Source: three-view drawing plus pictorial views. Frame: mm from the lowest corner of the part. Coordinates: 2 decimals unless noted, no trailing zeros. Order: outer loops, then holes, each group sorted by start corner. A loop starts at its lowest first (then second) coordinate and runs counter-clockwise, first axis right, second up. Notation, with made-up numbers: M 30.25,11 L 64.25,11 A18 cw 64.25,20 Z; hole C -17.75,-7 d4. An arc over 180 degrees is marked long. Use CSV: the item, a comma, the result in double quotes. Start each with the question number.
Q1. Section query A-A, the plane z = 11.5. State how many separate pieces and enclosed holes the cut face has, and give its area (3 significant figures).
Q2. Ray query, probe 1 along Y at (x, z) = (62, 16.75); probe 2 along Z at (x, y) = (37, 114). Return the intervals inside material, ascending.
Q3. Section query B-B, the plane x = 69. Output: boundary loops of the cut face in (y, z), and give its area (3 significant figures).
Q4. First-contact query: P1, Ø8, axis at x = 58, y = 24, coming from the +Z side; P2, Ø8, axis at y = 30, z = 8, coming from the -X side. Flat tips, straight axial feed; report the tip coordinate or a pass-through.
Q5. Section query C-C, the plane y = 60. Output: boundary loops of the cut face in (x, z).
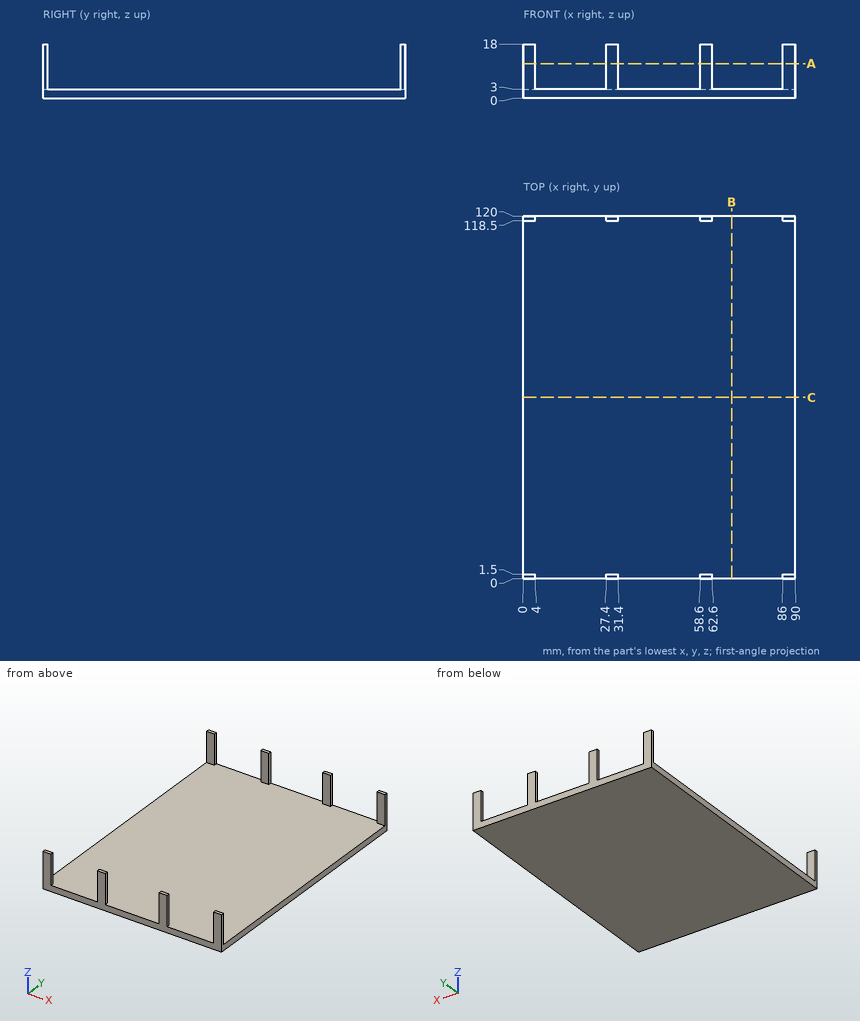
Responses:
1,separate pieces,"8"
1,enclosed holes,"0"
1,area,"48.0 mm²"
2,probe 1,"y = 0 to 1.5, 118.5 to 120"
2,probe 2,"z = 0 to 3"
3,outline,"M 0,0 L 120,0 L 120,3 L 0,3 Z"
3,area,"360 mm²"
4,P1,"stops at z = 3"
4,P2,"passes through"
5,outline,"M 0,0 L 90,0 L 90,3 L 0,3 Z"
